from build123d import *

# Parameters (mm, degrees)
F0_W          = 45
F0_H          = 20
F1_DEPTH      = 10
F1_DEPTH_BACK = 10
F2_R          = 3
F3_DEPTH      = 45.001
F4_R          = 1.5
F5_DEPTH      = 20.001
F6_R          = 1.5
F7_DEPTH      = 11.4029238886
F8_R          = 3
F9_DEPTH      = 4
F10_R         = 1.5
F11_DEPTH     = 3.4029238886


with BuildPart() as f1:
    # F0 (on Front) → F1 (new body, two sides)
    with BuildSketch(Plane.XZ) as f1_sk:
        Rectangle(F0_W, F0_H)
    extrude(amount=F1_DEPTH)
    extrude(f1_sk.sketch, amount=-F1_DEPTH_BACK)

    # F2 (on face) → F3 (cut, through all)
    with BuildSketch(Plane(origin=(-22.5, 0, 0), x_dir=(0, -1, 0), z_dir=(-1, 0, 0))):
        with Locations((-4, 0)):
            Circle(F2_R)
    extrude(amount=-F3_DEPTH, mode=Mode.SUBTRACT)

    # F4 (on face) → F5 (cut, through all)
    with BuildSketch(Plane.XZ.offset(10)):
        with Locations((19.5, 7)):
            Circle(F4_R)
        with Locations((2.5, -7)):
            Circle(F4_R)
    extrude(amount=-F5_DEPTH, mode=Mode.SUBTRACT)

    # F6 (on face) → F7 (cut, through all)
    with BuildSketch(Plane.XZ.offset(10)):
        with Locations((14.5, 0)):
            Circle(F6_R)
    extrude(amount=-F7_DEPTH, mode=Mode.SUBTRACT)

    # F8 (on face) → F9 (cut)
    with BuildSketch(Plane.XY.offset(10)):
        with Locations((2.5, 4)):
            Circle(F8_R)
    extrude(amount=-F9_DEPTH, mode=Mode.SUBTRACT)

    # F10 (on face) → F11 (cut, through all)
    with BuildSketch(Plane.XY.offset(6)):
        with Locations((2.5, 4)):
            Circle(F10_R)
    extrude(amount=-F11_DEPTH, mode=Mode.SUBTRACT)


solid = f1.part
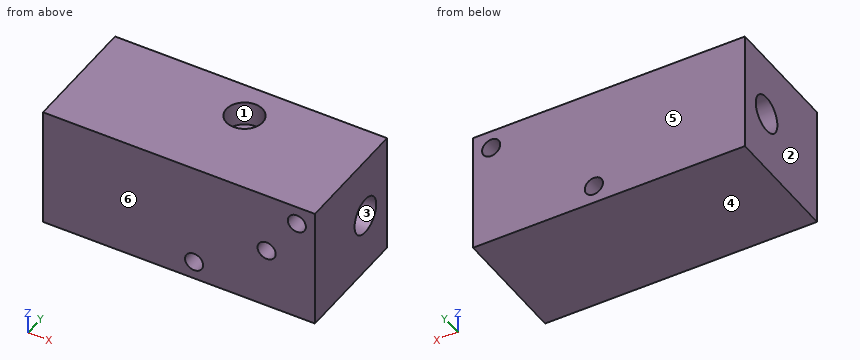
Read the model definition and answer for the solid it produces. Units are mm, in the model's axes. Face numbers are marked on the shaded views. A direction names the side the tool comes from. Coordinates: 2 decimals unless noted, no trailing zeros. Loops run counter-clockwise (first coordinate to the right, second up) from the corner with the lowest first, then second, coordinate; pieces in that order, holes last.
Q1. The part is cut by section B-B on y = -7.25. Write down the section's boundary in (x, z).
Q2. The part is cut by section C-C on z = 7. Write down the section's boundary in (x, y), and give its area (3 significant figures).
Q3. Each of these flat-tipped pins is pushed along its axis until it touches: pin 1 Ø3 at (x, y) = (3.5, 5) entering from +Z; pin 2 Ø3.5 at (x, z) = (14.5, 0) entering from -Y; pin 3 Ø2.5 at (x, y) = (2.5, 4) entering from +Z. Where does it stop, or does it pass through?
Q4. Which of the six approach directions +Z, -Z, +X, -X, +Y, -Y give full straight-line access (tool end or side, diameter ignored) to the marked faces 1 and 2?
Q5. The mould has two halves that part along Y. Classify the marked faces 3, 4, 5 and 6: +Y half, -Y half, draft (parallel to the pull), parting line (faces both ways), or undercut.
Q6. The part is cut by section D-D on x = 14.5. Write down the section's boundary in (y, z), and give its area (3 significant figures).
Q7. The part is cut by section A-A on z = -7. Write down the section's boundary in (x, y), and give its area (3 significant figures).
Q8. Consider probe 1 along Z at (x, y) = (-5.5, 4); probe 2 along Y at (x, z) = (2.5, 7); probe 3 along Z at (x, y) = (19.5, -5.5). Determine where each line is inside the solid, lowest interval first.
Results below:
1. outline: (-22.5, -10) - (22.5, -10) - (22.5, 10) - (-22.5, 10) - close; hole circle Ø3 at (2.5, -7); hole circle Ø3 at (14.5, 0); hole circle Ø3 at (19.5, 7)
2. outline: (-22.5, -10) - (18, -10) - (18, 10) - (-22.5, 10) - close; (21, -10) - (22.5, -10) - (22.5, 10) - (21, 10) - close; hole circle Ø6 at (2.5, 4)
2. area: 812 mm2
3. pin 1: stops at z = 6
3. pin 2: stops at y = -10
3. pin 3: stops at z = -2.73
4. face 1: +Z
4. face 2: +Z, -Z, -X, +Y, -Y
5. face 3: undercut
5. face 4: draft
5. face 5: +Y half
5. face 6: -Y half
6. outline: (-10, -10) - (10, -10) - (10, 10) - (-10, 10) - (-10, 1.5) - (1.4, 1.5) arc R3 cw (long way) to (1.4, -1.5) - (-10, -1.5) - close
6. area: 338 mm2
7. outline: (-22.5, -10) - (1, -10) - (1, 10) - (-22.5, 10) - close; (4, -10) - (22.5, -10) - (22.5, 10) - (4, 10) - close
7. area: 840 mm2
8. probe 1: z = -10 to -3, 3 to 10
8. probe 2: y = -10 to 1, 7 to 10
8. probe 3: z = -10 to 5.5, 8.5 to 10
